from build123d import *

# Parameters (mm, degrees)
SKETCH1_W           = 30
SKETCH1_H           = 30
SKETCH1_R           = 1.5
BOSS_EXTRUDE2_DEPTH = 0.9
SKETCH9_W           = 1
SKETCH9_H           = 24
BOSS_EXTRUDE3_DEPTH = 27
SKETCH10_R          = 12
BOSS_EXTRUDE4_DEPTH = 30
SKETCH11_R          = 12.5
BOSS_EXTRUDE5_DEPTH = 16.5
SKETCH12_R          = 4
BOSS_EXTRUDE6_DEPTH = 6.5
SKETCH13_R          = 2
BOSS_EXTRUDE7_DEPTH = 10
CUT_EXTRUDE1_START  = -8
CUT_EXTRUDE1_DEPTH  = 8


with BuildPart() as part:
    # Sketch1 → Boss-Extrude2 (new body)
    with BuildSketch(Plane(origin=(0, 0, 0), x_dir=(1, 0, 0), z_dir=(0, 1, 0))):
        Rectangle(SKETCH1_W, SKETCH1_H)
        with Locations(Location((-12, 12, 0), (0, 0, 270))):
            Circle(SKETCH1_R, mode=Mode.SUBTRACT)
        with Locations(Location((12, 12, 0), (0, 0, 270))):
            Circle(SKETCH1_R, mode=Mode.SUBTRACT)
        with Locations(Location((12, -12, 0), (0, 0, 270))):
            Circle(SKETCH1_R, mode=Mode.SUBTRACT)
        with Locations(Location((-12, -12, 0), (0, 0, 270))):
            Circle(SKETCH1_R, mode=Mode.SUBTRACT)
    extrude(amount=BOSS_EXTRUDE2_DEPTH)

    # Sketch9 → Boss-Extrude3 (add)
    with BuildSketch(Plane(origin=(0, 0, 0), x_dir=(1, 0, 0), z_dir=(0, 1, 0))):
        with Locations((-15.5, 0)):
            Rectangle(SKETCH9_W, SKETCH9_H)
    extrude(amount=BOSS_EXTRUDE3_DEPTH)

    # Sketch10 → Boss-Extrude4 (add)
    with BuildSketch(Plane(origin=(-15, 0, 0), x_dir=(0, 0, -1), z_dir=(1, 0, 0))):
        with Locations(Location((0, 14.5, 0), (0, 0, 180))):
            Circle(SKETCH10_R)
    extrude(amount=BOSS_EXTRUDE4_DEPTH)

    # Sketch11 → Boss-Extrude5 (add)
    with BuildSketch(Plane.ZY.offset(16)):
        with Locations(Location((0, 14.5, 0), (0, 0, 163.739795292))):
            Circle(SKETCH11_R)
    extrude(amount=BOSS_EXTRUDE5_DEPTH)

    # Sketch12 → Boss-Extrude6 (add)
    with BuildSketch(Plane.ZY.offset(32.5)):
        with Locations(Location((0, 14.5, 0), (0, 0, 180))):
            Circle(SKETCH12_R)
    extrude(amount=BOSS_EXTRUDE6_DEPTH)

    # Sketch13 → Boss-Extrude7 (add)
    with BuildSketch(Plane.ZY.offset(39)):
        with Locations((0, 14.5)):
            Circle(SKETCH13_R)
    extrude(amount=BOSS_EXTRUDE7_DEPTH)

    # Sketch14 → Cut-Extrude1 (cut)
    with BuildSketch(Plane.ZY.offset(49).offset(CUT_EXTRUDE1_START)):
        with BuildLine():
            Line((-1.322875656, 16), (1.322875656, 16))
            ThreePointArc((1.322875656, 16), (0, 16.5), (-1.322875656, 16))
        make_face()
    extrude(amount=CUT_EXTRUDE1_DEPTH, mode=Mode.SUBTRACT)


solid = part.part
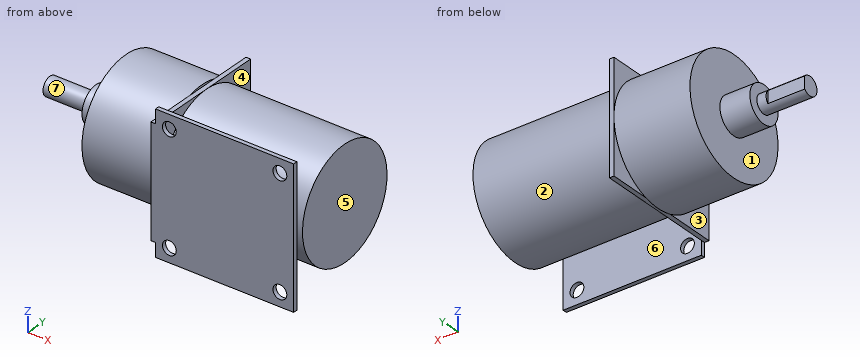
Here's how the part is built. I have some questions about the finished solid (model axes, mm). Face numbers are marked on the shaded views. A direction names the side the tool comes from. Coordinates: 2 decimals unless noted, no trailing zeros. Write each loop counter-clockwise with the first axis right and the second up, starting at its lowest first coordinate (ties: lowest second). Pieces come first, ordered by that corner, then holes.
Item 1: If we mould it in two halves opening along Y, with no side actions, what happens to the marked faces 5, 6 and 7? For each: +Y half, -Y half, draft (parallel to the pull), parting line (faces both ways), or undercut.
Item 2: On a 3-axis mill with a long thin cutter (end or side, diameter ignored), from which of +Z, -Z, +X, -X, +Y, -Y can I reach the whole of each face in a straight line? I mean the marked faces 1, 2, 3 and 4. Say none if no direction works.
Item 3: I want a section at A-A on x = -6. Write out the boundary of the cut face in (y, z), and give its area (3 significant figures).
Item 4: I want a section at D-D on y = 20. Write out the boundary of the cut face in (x, z), and give its area (3 significant figures).
Item 5: I want a section at B-B on x = 12. Write out the boundary of the cut face in (y, z), and give its area (3 significant figures).
Item 6: I want a section at C-C on z = -7.5. Write out the boundary of the cut face in (x, y).
Item 7: Will these pins go through, and if not, where does the flat tip stop? pin 1 (6 mm diameter, centred on x = -34, y = 13.5, fed in from -Z); pin 2 (1.1 mm diameter, centred on x = -15.5, y = 19, fed in from +Z); pin 3 (2.5 mm diameter, centred on x = -12, z = 12, fed in from +Y); pin 4 (5 mm diameter, centred on x = -12, z = -12, fed in from -Y).
Item 8: If I drill on line 1 (X direction, y = 6.25, z = 2.5); line 2 (X direction, y = 26, z = -11.25); line 3 (Y direction, x = 6, z = 4), over which ranges is the centre line in solid material (lowest first)?
Findings below:
1. face 5: draft
1. face 6: undercut
1. face 7: parting line
2. face 1: -X
2. face 2: +X
2. face 3: -X, -Y
2. face 4: +X, +Y
3. outline: (0, -15) - (0.9, -15) - (0.9, 15) - (0, 15) - close; circle Ø24 at (14.5, 0)
3. area: 479 mm2
4. outline: (-32.5, -11.22) - (-16, -11.22) - (-16, -12) - (-15, -12) - (-15, -10.67) - (15, -10.67) - (15, 10.67) - (-15, 10.67) - (-15, 12) - (-16, 12) - (-16, 11.22) - (-32.5, 11.22) - close
4. area: 1,030 mm2
5. outline: (0, -15) - (0.9, -15) - (0.9, -13.5) - (0, -13.5) - close; (0, -10.5) - (0.9, -10.5) - (0.9, 10.5) - (0, 10.5) - close; (0, 13.5) - (0.9, 13.5) - (0.9, 15) - (0, 15) - close; circle Ø24 at (14.5, 0)
5. area: 474 mm2
6. outline: (-32.5, 4.5) - (-16, 4.5) - (-16, 0) - (15, 0) - (15, 0.9) - (-15, 0.9) - (-15, 5.13) - (15, 5.13) - (15, 23.87) - (-15, 23.87) - (-15, 27) - (-16, 27) - (-16, 24.5) - (-32.5, 24.5) - close
7. pin 1: stops at z = -12.5
7. pin 2: stops at z = 12
7. pin 3: stops at y = 19.83
7. pin 4: stops at y = 0
8. line 1: x = -32.5 to 15
8. line 2: x = -16 to -15
8. line 3: y = 0 to 0.9, 3.19 to 25.81
